The listing builds one solid part. Answer for the finished solid, in the listing's coordinates (mm). A direction names the side the tool comes from. Coordinates: 2 decimals unless noted, no trailing zeros. Order: outer loops, then holes, each group sorted by start corner. A loop starts at its lowest first (then second) coordinate and runs counter-clockwise, first axis right, second up.
```python
from build123d import *

# Parameters (mm, degrees)
F1_DEPTH = 10


with BuildPart() as f1:
    # F0 (on Front) → F1 (new body)
    with BuildSketch(Plane.XZ):
        Polygon((0, 90), (0, 0), (20, 0), (20, 30), (20, 75.879364), (117.741286, 75.879364), (117.741286, 0), (137.741286, 0), (137.741286, 75.879364), (235.482572, 75.879364), (235.482572, 30), (235.482572, 0), (255.482572, 0), (255.482572, 180), (235.482572, 180), (235.482572, 115.879364), (137.741286, 115.879364), (137.741286, 179.137096), (127.741286, 179.137096), (117.741286, 179.137096), (117.741286, 115.879364), (20, 115.879364), (20, 180), (0, 180), (0, 115.879364), align=None)
    extrude(amount=F1_DEPTH)


solid = f1.part
```
1) A cutting plane is placed at B-B, the plane y = -2. Write down the section's boundary in (x, z).
2) A cutting plane is placed at A-A, the plane z = 21. Write down the section's boundary in (x, y).
3) Straight lines are drawn through the part: probe 1 along X at (y, z) = (-4, 30); probe 2 along Z at (x, y) = (175, -1.5). For each, find the intervals that lie inside material, in ascending order.
4) A cutting plane is placed at C-C, the plane x = 59.5. Write down the section's boundary in (y, z).
5) For faces 4 (the flat face through (128, -5, 179.137)), 5 (the flat face through (246, -5, 180)), 6 (the flat face through (20, -5, 37)), determine the directions among +Z, -Z, +X, -X, +Y, -Y from which every point of the face is accessible in a straight line to the end or side of a thin tool.
6) Each of these flat-tipped pins is pushed along its axis until it touches: P1, Ø3, axis at x = 85, y = -4.5, coming from the +Z side; P2, Ø3, axis at x = 85.5, y = -6, coming from the -Z side; P3, Ø5, axis at x = 126, y = -3, coming from the +Z side. Where does it stop, or does it pass through?
7) The mould has two halves that part along X. Classify faces 1 (the flat face through (235.483, -5, 38)), 2 (the flat face through (126, -10, 91)), 3 (the flat face through (255.483, -5, 89)): released by +X, released by -X, zero draft, split by the parting line, or undercut.
Working result:
1. outline: (0, 0) - (20, 0) - (20, 75.88) - (117.74, 75.88) - (117.74, 0) - (137.74, 0) - (137.74, 75.88) - (235.48, 75.88) - (235.48, 0) - (255.48, 0) - (255.48, 180) - (235.48, 180) - (235.48, 115.88) - (137.74, 115.88) - (137.74, 179.14) - (117.74, 179.14) - (117.74, 115.88) - (20, 115.88) - (20, 180) - (0, 180) - close
2. outline: (0, -10) - (20, -10) - (20, 0) - (0, 0) - close; (117.74, -10) - (137.74, -10) - (137.74, 0) - (117.74, 0) - close; (235.48, -10) - (255.48, -10) - (255.48, 0) - (235.48, 0) - close
3. probe 1: x = 0 to 20, 117.74 to 137.74, 235.48 to 255.48
3. probe 2: z = 75.88 to 115.88
4. outline: (-10, 75.88) - (0, 75.88) - (0, 115.88) - (-10, 115.88) - close
5. face 4: +Z, +Y, -Y
5. face 5: +Z, +X, -X, +Y, -Y
5. face 6: -Z, +Y, -Y
6. P1: stops at z = 115.88
6. P2: stops at z = 75.88
6. P3: stops at z = 179.14
7. face 1: undercut
7. face 2: zero draft
7. face 3: released by +X
